from build123d import *

# Parameters (mm, degrees)
F0_W     = 419.1
F0_H     = 552.45
F0_R     = 3.96875
F1_DEPTH = 3.175


with BuildPart() as f1:
    # F0 (on Top) → F1 (new body)
    with BuildSketch(Plane.XY):
        with Locations((209.55, 276.225)):
            Rectangle(F0_W, F0_H)
        with Locations((9.454559, 9.666916)):
            Circle(F0_R, mode=Mode.SUBTRACT)
        with BuildLine():
            Line((133.35, 12.84139), (19.05, 12.84139))
            ThreePointArc((19.05, 12.84139), (14.559872, 14.701262), (12.7, 19.19139))
            Line((12.7, 19.19139), (12.7, 133.49139))
            ThreePointArc((12.7, 133.49139), (14.559872, 137.981518), (19.05, 139.84139))
            Line((19.05, 139.84139), (133.35, 139.84139))
            ThreePointArc((133.35, 139.84139), (137.840128, 137.981518), (139.7, 133.49139))
            Line((139.7, 133.49139), (139.7, 19.19139))
            ThreePointArc((139.7, 19.19139), (137.840128, 14.701262), (133.35, 12.84139))
        make_face(mode=Mode.SUBTRACT)
        with Locations((142.804305, 9.666916)):
            Circle(F0_R, mode=Mode.SUBTRACT)
        with BuildLine():
            Line((272.979305, 133.420695), (272.979305, 19.120695))
            ThreePointArc((272.979305, 19.120695), (271.119433, 14.630567), (266.629305, 12.770695))
            Line((266.629305, 12.770695), (152.329305, 12.770695))
            ThreePointArc((152.329305, 12.770695), (147.839177, 14.630567), (145.979305, 19.120695))
            Line((145.979305, 19.120695), (145.979305, 133.420695))
            ThreePointArc((145.979305, 133.420695), (147.839177, 137.910823), (152.329305, 139.770695))
            Line((152.329305, 139.770695), (266.629305, 139.770695))
            ThreePointArc((266.629305, 139.770695), (271.119433, 137.910823), (272.979305, 133.420695))
        make_face(mode=Mode.SUBTRACT)
        with Locations((9.454559, 142.945695)):
            Circle(F0_R, mode=Mode.SUBTRACT)
        with Locations((9.454559, 276.224473)):
            Circle(F0_R, mode=Mode.SUBTRACT)
        with BuildLine():
            Line((139.629305, 266.770695), (139.629305, 152.470695))
            ThreePointArc((139.629305, 152.470695), (137.769433, 147.980567), (133.279305, 146.120695))
            Line((133.279305, 146.120695), (18.979305, 146.120695))
            ThreePointArc((18.979305, 146.120695), (14.489177, 147.980567), (12.629305, 152.470695))
            Line((12.629305, 152.470695), (12.629305, 266.770695))
            ThreePointArc((12.629305, 266.770695), (14.489177, 271.260823), (18.979305, 273.120695))
            Line((18.979305, 273.120695), (133.279305, 273.120695))
            ThreePointArc((133.279305, 273.120695), (137.769433, 271.260823), (139.629305, 266.770695))
        make_face(mode=Mode.SUBTRACT)
        with Locations((142.804305, 142.945695)):
            Circle(F0_R, mode=Mode.SUBTRACT)
        with Locations((142.804305, 276.224473)):
            Circle(F0_R, mode=Mode.SUBTRACT)
        with Locations((276.154051, 9.666916)):
            Circle(F0_R, mode=Mode.SUBTRACT)
        with Locations((409.503797, 9.666916)):
            Circle(F0_R, mode=Mode.SUBTRACT)
        with BuildLine():
            Line((406.4, 133.35), (406.4, 19.05))
            ThreePointArc((406.4, 19.05), (404.540128, 14.559872), (400.05, 12.7))
            Line((400.05, 12.7), (285.75, 12.7))
            ThreePointArc((285.75, 12.7), (281.259872, 14.559872), (279.4, 19.05))
            Line((279.4, 19.05), (279.4, 133.35))
            ThreePointArc((279.4, 133.35), (281.259872, 137.840128), (285.75, 139.7))
            Line((285.75, 139.7), (400.05, 139.7))
            ThreePointArc((400.05, 139.7), (404.540128, 137.840128), (406.4, 133.35))
        make_face(mode=Mode.SUBTRACT)
        with Locations((276.154051, 142.945695)):
            Circle(F0_R, mode=Mode.SUBTRACT)
        with BuildLine():
            Line((273.05, 266.84139), (273.05, 152.54139))
            ThreePointArc((273.05, 152.54139), (271.190128, 148.051262), (266.7, 146.19139))
            Line((266.7, 146.19139), (152.4, 146.19139))
            ThreePointArc((152.4, 146.19139), (147.909872, 148.051262), (146.05, 152.54139))
            Line((146.05, 152.54139), (146.05, 266.84139))
            ThreePointArc((146.05, 266.84139), (147.909872, 271.331518), (152.4, 273.19139))
            Line((152.4, 273.19139), (266.7, 273.19139))
            ThreePointArc((266.7, 273.19139), (271.190128, 271.331518), (273.05, 266.84139))
        make_face(mode=Mode.SUBTRACT)
        with Locations((276.154051, 276.224473)):
            Circle(F0_R, mode=Mode.SUBTRACT)
        with Locations((409.503797, 142.945695)):
            Circle(F0_R, mode=Mode.SUBTRACT)
        with BuildLine():
            Line((406.4, 266.7), (406.4, 152.4))
            ThreePointArc((406.4, 152.4), (404.540128, 147.909872), (400.05, 146.05))
            Line((400.05, 146.05), (285.75, 146.05))
            ThreePointArc((285.75, 146.05), (281.259872, 147.909872), (279.4, 152.4))
            Line((279.4, 152.4), (279.4, 266.7))
            ThreePointArc((279.4, 266.7), (281.259872, 271.190128), (285.75, 273.05))
            Line((285.75, 273.05), (400.05, 273.05))
            ThreePointArc((400.05, 273.05), (404.540128, 271.190128), (406.4, 266.7))
        make_face(mode=Mode.SUBTRACT)
        with Locations((409.503797, 276.224473)):
            Circle(F0_R, mode=Mode.SUBTRACT)
        with BuildLine():
            Line((139.7, 400.05), (139.7, 285.75))
            ThreePointArc((139.7, 285.75), (137.840128, 281.259872), (133.35, 279.4))
            Line((133.35, 279.4), (19.05, 279.4))
            ThreePointArc((19.05, 279.4), (14.559872, 281.259872), (12.7, 285.75))
            Line((12.7, 285.75), (12.7, 400.05))
            ThreePointArc((12.7, 400.05), (14.559872, 404.540128), (19.05, 406.4))
            Line((19.05, 406.4), (133.35, 406.4))
            ThreePointArc((133.35, 406.4), (137.840128, 404.540128), (139.7, 400.05))
        make_face(mode=Mode.SUBTRACT)
        with Locations((9.454559, 409.503252)):
            Circle(F0_R, mode=Mode.SUBTRACT)
        with Locations((142.804305, 409.503252)):
            Circle(F0_R, mode=Mode.SUBTRACT)
        with BuildLine():
            Line((139.7, 533.4), (139.7, 419.1))
            ThreePointArc((139.7, 419.1), (137.840128, 414.609872), (133.35, 412.75))
            Line((133.35, 412.75), (19.05, 412.75))
            ThreePointArc((19.05, 412.75), (14.559872, 414.609872), (12.7, 419.1))
            Line((12.7, 419.1), (12.7, 533.4))
            ThreePointArc((12.7, 533.4), (14.559872, 537.890128), (19.05, 539.75))
            Line((19.05, 539.75), (133.35, 539.75))
            ThreePointArc((133.35, 539.75), (137.840128, 537.890128), (139.7, 533.4))
        make_face(mode=Mode.SUBTRACT)
        with Locations((9.454559, 542.78203)):
            Circle(F0_R, mode=Mode.SUBTRACT)
        with Locations((142.804305, 542.78203)):
            Circle(F0_R, mode=Mode.SUBTRACT)
        with BuildLine():
            Line((273.050001, 400.05), (273.050001, 285.75))
            ThreePointArc((273.050001, 285.75), (271.190129, 281.259872), (266.700001, 279.4))
            Line((266.700001, 279.4), (152.400001, 279.4))
            ThreePointArc((152.400001, 279.4), (147.909873, 281.259872), (146.050001, 285.75))
            Line((146.050001, 285.75), (146.050001, 400.05))
            ThreePointArc((146.050001, 400.05), (147.909873, 404.540128), (152.400001, 406.4))
            Line((152.400001, 406.4), (266.700001, 406.4))
            ThreePointArc((266.700001, 406.4), (271.190129, 404.540128), (273.050001, 400.05))
        make_face(mode=Mode.SUBTRACT)
        with Locations((276.154051, 409.503252)):
            Circle(F0_R, mode=Mode.SUBTRACT)
        with BuildLine():
            Line((406.4, 400.05), (406.4, 285.75))
            ThreePointArc((406.4, 285.75), (404.540128, 281.259872), (400.05, 279.4))
            Line((400.05, 279.4), (285.75, 279.4))
            ThreePointArc((285.75, 279.4), (281.259872, 281.259872), (279.4, 285.75))
            Line((279.4, 285.75), (279.4, 400.05))
            ThreePointArc((279.4, 400.05), (281.259872, 404.540128), (285.75, 406.4))
            Line((285.75, 406.4), (400.05, 406.4))
            ThreePointArc((400.05, 406.4), (404.540128, 404.540128), (406.4, 400.05))
        make_face(mode=Mode.SUBTRACT)
        with Locations((409.503797, 409.503252)):
            Circle(F0_R, mode=Mode.SUBTRACT)
        with BuildLine():
            Line((273.05, 533.4), (273.05, 419.1))
            ThreePointArc((273.05, 419.1), (271.190128, 414.609872), (266.7, 412.75))
            Line((266.7, 412.75), (152.4, 412.75))
            ThreePointArc((152.4, 412.75), (147.909872, 414.609872), (146.05, 419.1))
            Line((146.05, 419.1), (146.05, 533.4))
            ThreePointArc((146.05, 533.4), (147.909872, 537.890128), (152.4, 539.75))
            Line((152.4, 539.75), (266.7, 539.75))
            ThreePointArc((266.7, 539.75), (271.190128, 537.890128), (273.05, 533.4))
        make_face(mode=Mode.SUBTRACT)
        with Locations((276.154051, 542.78203)):
            Circle(F0_R, mode=Mode.SUBTRACT)
        with BuildLine():
            Line((406.4, 533.4), (406.4, 419.1))
            ThreePointArc((406.4, 419.1), (404.540128, 414.609872), (400.05, 412.75))
            Line((400.05, 412.75), (285.75, 412.75))
            ThreePointArc((285.75, 412.75), (281.259872, 414.609872), (279.4, 419.1))
            Line((279.4, 419.1), (279.4, 533.4))
            ThreePointArc((279.4, 533.4), (281.259872, 537.890128), (285.75, 539.75))
            Line((285.75, 539.75), (400.05, 539.75))
            ThreePointArc((400.05, 539.75), (404.540128, 537.890128), (406.4, 533.4))
        make_face(mode=Mode.SUBTRACT)
        with Locations((409.503797, 542.78203)):
            Circle(F0_R, mode=Mode.SUBTRACT)
    extrude(amount=F1_DEPTH)


solid = f1.part
CAD build for the part. Positions are in the model's coordinates, mm. Round coordinates to 2 decimals unless told otherwise and drop trailing zeros. Write each loop counter-clockwise with the first axis right and the second up, starting at its lowest first coordinate (ties: lowest second). Pieces come first, ordered by that corner, then holes. Notation, with made-up numbers: M 66,65 L 87,65 A24 cw 87,97 Z; hole C 30.25,46 d1. An arc over 180 degrees is marked long. Put each result on its own line as item: value. Start each with the question number.
1) Pin check, flat tip, straight feed: pin 1 Ø10 at (x, y) = (288, 59) entering from -Z (1 decimal). Stop position of the tip, or through.
2) Drill centre lines: probe 1 along X at (y, z) = (311, 2.7); probe 2 along Y at (x, z) = (47, 1.8); probe 3 along X at (y, z) = (212, 2.25). Where is each one in solid material? Low to high. Write a range as [from, to].
3) Saw through at C-C, the plane z = 2. Count the separate pieces of the cut face and the enclosed holes in it, and give its area (3 significant figures).
4) Saw through at A-A, the plane y = 43. Write the cut outline in (x, z) (3 decimals).
5) Saw through at B-B, the plane x = 45.5. Write the cut outline in (y, z) (3 decimals), and give its area (3 significant figures).
Resolved:
1. pin 1: through
2. probe 1: [0, 12.7], [139.7, 146.05], [273.05, 279.4], [406.4, 419.1]
2. probe 2: [0, 12.84], [139.84, 146.12], [273.12, 279.4], [406.4, 412.75], [539.75, 552.45]
2. probe 3: [0, 12.63], [139.63, 146.05], [273.05, 279.4], [406.4, 419.1]
3. separate pieces: 1
3. enclosed holes: 32
3. area: 37,400 mm²
4. outline: M 0,0 L 12.7,0 L 12.7,3.175 L 0,3.175 Z; M 139.7,0 L 145.979,0 L 145.979,3.175 L 139.7,3.175 Z; M 272.979,0 L 279.4,0 L 279.4,3.175 L 272.979,3.175 Z; M 406.4,0 L 419.1,0 L 419.1,3.175 L 406.4,3.175 Z
5. outline: M 0,0 L 12.841,0 L 12.841,3.175 L 0,3.175 Z; M 139.841,0 L 146.121,0 L 146.121,3.175 L 139.841,3.175 Z; M 273.121,0 L 279.4,0 L 279.4,3.175 L 273.121,3.175 Z; M 406.4,0 L 412.75,0 L 412.75,3.175 L 406.4,3.175 Z; M 539.75,0 L 552.45,0 L 552.45,3.175 L 539.75,3.175 Z
5. area: 141 mm²
